```python
from build123d import *

# Parameters (mm, degrees)
F1_DEPTH = 4
F2_W     = 15.7914069632
F2_H     = 4
F3_DEPTH = 7
F6_W     = 13.4452040827
F6_H     = 2.2
F7_DEPTH = 8
F8_DEPTH = 14.5045625426


with BuildPart() as f1:
    # F0 (on Top) → F1 (new body, symmetric)
    with BuildSketch(Plane.XY):
        with BuildLine():
            ThreePointArc((40.1879624894, -7.1882514277), (41.8101711711, -7.1412327294), (43.3619882248, -7.6162438838))
            ThreePointArc((43.3619882248, -7.6162438838), (55.6359555142, 0), (43.3619882248, 7.6162438838))
            ThreePointArc((43.3619882248, 7.6162438838), (41.8101711711, 7.1412327294), (40.1879624894, 7.1882514277))
            Line((40.1879624894, 7.1882514277), (2.3847180591, 14.5364577665))
            ThreePointArc((2.3847180591, 14.5364577665), (0.4038763846, 14.2404189947), (-0.9492234874, 12.7637696016))
            Line((-0.9492234874, 12.7637696016), (-3.9139870299, 5.7792243959))
            Line((-3.9139870299, 5.7792243959), (0.6885372374, 3.8255687534))
            Line((0.6885372374, 3.8255687534), (2.0712616343, 7.0830632951))
            ThreePointArc((2.0712616343, 7.0830632951), (3.4243615063, 8.5597126882), (5.4052031808, 8.85575146))
            Line((5.4052031808, 8.85575146), (39.8374709782, 2.1627966012))
            ThreePointArc((39.8374709782, 2.1627966012), (42.1235130158, 2.251618892), (44.1306946704, 3.3493890877))
            ThreePointArc((44.1306946704, 3.3493890877), (51.6359555142, 0), (44.1306946704, -3.3493890877))
            ThreePointArc((44.1306946704, -3.3493890877), (42.1235130158, -2.251618892), (39.8374709782, -2.1627966012))
            Line((39.8374709782, -2.1627966012), (4.6474579448, -9.0030422132))
            ThreePointArc((4.6474579448, -9.0030422132), (2.8309512307, -8.7880444755), (1.4769547473, -7.5581606629))
            Line((1.4769547473, -7.5581606629), (-9.963304434, 12.256949491))
            ThreePointArc((-9.963304434, 12.256949491), (-14.5143086091, 9.879543395), (-18.655423863, 6.8439440802))
            ThreePointArc((-18.655423863, 6.8439440802), (-21.653397971, 4.0115098086), (-24.3606178303, 0.9))
            Line((-24.3606178303, 0.9), (-22.5606178303, -0.9))
            Line((-22.5606178303, -0.9), (-20.7606178303, 0.9))
            Line((-20.7606178303, 0.9), (-18.9606178303, -0.9))
            Line((-18.9606178303, -0.9), (-17.1606178303, 0.9))
            Line((-17.1606178303, 0.9), (-15.3606178303, -0.9))
            Line((-15.3606178303, -0.9), (-13.5606178303, 0.9))
            Line((-13.5606178303, 0.9), (-11.7606178303, -0.9))
            Line((-11.7606178303, -0.9), (-9.9606178303, 0.9))
            Line((-9.9606178303, 0.9), (-9.4656430834, 1.3949747468))
            Line((-9.4656430834, 1.3949747468), (-1.0699396018, -13.1468102486))
            ThreePointArc((-1.0699396018, -13.1468102486), (0.2840568815, -14.3766940612), (2.1005635956, -14.5916917989))
            Line((2.1005635956, -14.5916917989), (40.1879624894, -7.1882514277))
        make_face()
    extrude(amount=F1_DEPTH, both=True)

    # F2 (on face) → F3 (cut)
    with BuildSketch(Plane(origin=(-6.4951905284, -3.75, 0), x_dir=(0.5, -0.8660254038, 0), z_dir=(-0.8660254038, -0.5, 0))):
        with Locations((1.9547983715, 0)):
            Rectangle(F2_W, F2_H)
    extrude(amount=-F3_DEPTH, mode=Mode.SUBTRACT)

    # F6 (on face) → F7 (cut)
    with BuildSketch(Plane(origin=(6.2177817942, 3.306053224, 0), x_dir=(0.4694715628, -0.8829475929, 0), z_dir=(-0.8829475929, -0.4694715628, 0))):
        with Locations((-9.7771301106, -2.9)):
            Rectangle(F6_W, F6_H)
        with Locations((-9.7771301106, 2.9)):
            Rectangle(F6_W, F6_H)
    extrude(amount=F7_DEPTH, mode=Mode.SUBTRACT)

    # F8 (add, up to face): a face of the model
    f8_faces = [f1.faces().sort_by_distance(p)[0] for p in [
        (-1.6127248962, 4.8023965747, 0),
    ]]


with BuildPart() as f1b:
    # F0 (on Top) → F1, piece 2 (new body, symmetric)
    with BuildSketch(Plane.XY):
        with BuildLine():
            ThreePointArc((-18.655423863, -7.7815652767), (-10.0426174907, -12.2242484166), (-0.8057885607, -15.1566294295))
            Line((-0.8057885607, -15.1566294295), (-9.9606178303, 0.7))
            Line((-9.9606178303, 0.7), (-11.7606178303, -1.1))
            Line((-11.7606178303, -1.1), (-13.5606178303, 0.7))
            Line((-13.5606178303, 0.7), (-15.3606178303, -1.1))
            Line((-15.3606178303, -1.1), (-17.1606178303, 0.7))
            Line((-17.1606178303, 0.7), (-18.9606178303, -1.1))
            Line((-18.9606178303, -1.1), (-20.7606178303, 0.7))
            Line((-20.7606178303, 0.7), (-22.5606178303, -1.1))
            Line((-22.5606178303, -1.1), (-24.3606178303, 0.7))
            Line((-24.3606178303, 0.7), (-24.3606178303, -3.443194404))
            ThreePointArc((-24.3606178303, -3.443194404), (-21.6051594937, -5.7401224515), (-18.655423863, -7.7815652767))
        make_face()
    extrude(amount=F1_DEPTH, both=True)


with BuildPart() as f1_1:
    add(f1.part)

    add(f1b.part)  # F8 merges F1b
    extrude(f8_faces, amount=F8_DEPTH)


solid = f1_1.part
```
CAD build for the part. Positions are in the model's coordinates, mm. A direction names the side the tool comes from. Round coordinates to 2 decimals unless told otherwise and drop trailing zeros. Order: outer loops, then holes, each group sorted by start corner. A loop starts at its lowest first (then second) coordinate and runs counter-clockwise, first axis right, second up. Notation, with made-up numbers: (8.25, 14) - (14.25, 14) arc R18 ccw to (14.25, 32) - close; hole circle Ø1 at (-26, 3.25). An arc over 180 degrees is marked (long way). Answer in a Markdown table with one row per item. Add a question column.
(1) Drop flat-ended pins along their axis: pin 1 Ø4 at (x, z) = (20, 0.5) entering from +Y; pin 2 Ø7 at (x, y) = (47.14, 0) entering from +Z; pin 3 Ø1.5 at (y, z) = (-1, 0.5) entering from +X; pin 4 Ø3.5 at (x, y) = (0.5, 4.5) entering from -Z. Give the stop position or say it passes through.
(2) Band-saw the part on B-B on x = 28. List the corners of the cut face in (y, z), and give its area (3 significant figures).
(3) Band-saw the part on C-C on y = 0. Count the separate pieces of the cut face and the enclosed holes in it, and give its area (3 significant figures).
(4) 3-axis set-ups, long thin cutter, end or side, ignore diameter. For faces 1 (the face through (41.833, 7.144, 0.056)), 2 (the face through (18.4, -6.5, 4)), 3 (the face through (20.88, -10.94, 0.06)), 4 (the face through (-3, 3, -1.8)), 5 (the face through (22.38, 5.556, 0.056)): which of +Z, -Z, +X, -X, +Y, -Y reach the whole face in a straight line?
(5) Band-saw the part on A-A on y = 11.25. List the corners of the cut face in (x, z).
(6) Probe L1, parallel to X at y = -1.75, z = 1.75; L2, parallel to Y at x = -3, z = 0.5; L3, parallel to Y at x = -4, z = 1. List the from-to ranges inside material, lowest first. Write a range as [from, to].
(7) Mould opens along X. For faces 6 (the face through (-21.645, -5.71, 0.056)), 7 (the face through (-13, -5, -4)), 8 (the face through (-3, 3, 1.8)) say: +X half, -X half, draft (parallel to the pull), parting line (faces both ways), or undercut.
Data:
| question | item | result |
|---|---|---|
| 1 | pin 1 | stops at y = 11.5 |
| 1 | pin 2 | passes through |
| 1 | pin 3 | stops at x = 55.63 |
| 1 | pin 4 | stops at z = -1.8 |
| 2 | outline | (-9.56, -4) - (-4.46, -4) - (-4.46, 4) - (-9.56, 4) - close; (4.46, -4) - (9.56, -4) - (9.56, 4) - (4.46, 4) - close |
| 2 | area | 81.5 mm^2 |
| 3 | separate pieces | 13 |
| 3 | enclosed holes | 0 |
| 3 | area | 180 mm^2 |
| 4 | face 1 | +Z, -Z, +Y |
| 4 | face 2 | +Z, +X, -X, +Y, -Y |
| 4 | face 3 | +Z, -Z, -Y |
| 4 | face 4 | none |
| 4 | face 5 | +Z, -Z |
| 5 | outline | (-12.1, -4) - (-9.38, -4) - (-9.38, 4) - (-12.1, 4) - close; (-1.59, -1.8) - (1.99, -1.8) - (1.99, -4) - (19.29, -4) - (19.29, 4) - (1.99, 4) - (1.99, 1.8) - (-1.59, 1.8) - close |
| 6 | L1 | x = [-24.36, -8.55], [-7.11, -1.68], [51.28, 55.45] |
| 6 | L2 | y = [-14.61, -11.36], [-4.86, 7.93] |
| 6 | L3 | y = [-14.34, -9.62], [-7.22, 5.58] |
| 7 | face 6 | -X half |
| 7 | face 7 | draft |
| 7 | face 8 | undercut |
